Read the model definition and answer for the solid it produces. Units are mm, in the model's axes. A direction names the side the tool comes from. Give positions to 0.01 mm unless a question says otherwise; leave off trailing zeros. Order: outer loops, then holes, each group sorted by start corner. A loop starts at its lowest first (then second) coordinate and runs counter-clockwise, first axis right, second up.
Item 1: Find the intervals of material crossed by line 1 along Y through (x, z) = (0, -5.5); line 2 along Y through (x, z) = (-10.25, 0.75); line 3 along Z through (x, y) = (-2, 28), in increasing order.
Item 2: Given pin 1 Ø5 at (x, y) = (0, 39) entering from -Z; pin 2 Ø2 at (y, z) = (108.5, 8) entering from +X, each flat-ended and moving along its own axis, determine where each tip first touches the part or whether it passes through.
Item 3: A cutting plane is placed at A-A (x = 0). State how many separate pieces and enclosed holes the cut face has, plus the area to 3 significant figures.
Item 4: A cutting plane is placed at B-B (y = 39). Write down the section's boundary in (x, z).
Item 5: A cutting plane is placed at C-C (y = 309.5). Write down the section's boundary in (x, z), plus the area to 3 significant figures.
Item 6: Which of the six approach directions +Z, -Z, +X, -X, +Y, -Y give full straight-line access (tool end or side, diameter ignored) to faces 4 (the face through (0, 22, -1)), 5 (the face through (0, 0, -4))?
Item 7: The mould has two halves that part along Y. Classify faces 1 (the face through (-1, 173, 10.1)), 2 (the face through (0, 0, 4)), 3 (the face through (-0.521, 18.466, -5.486)): +Y half, -Y half, draft (parallel to the pull), parting line (faces both ways), or undercut.
from build123d import *

# Parameters (mm, degrees)
F0_W      = 30
F0_H      = 20.2
F1_DEPTH  = 350
F2_R      = 5
F3_R      = 3
F4_W      = 45.5
F4_H      = 2
F5_DEPTH  = 30.001
F6_W      = 5
F6_H      = 5
F7_DEPTH  = 30.001
F8_R      = 4
F9_DEPTH  = 20.201
F10_DEPTH = 30.001


with BuildPart() as f1:
    # F0 (on Front) → F1 (new body)
    with BuildSketch(Plane.XZ):
        Rectangle(F0_W, F0_H)
    extrude(amount=-F1_DEPTH)

    # F2
    f2_edges = [f1.edges().sort_by_distance(p)[0] for p in [
        (15, 175, 10.1),
    ]]
    fillet(f2_edges, radius=F2_R)

    # F3
    f3_edges = [f1.edges().sort_by_distance(p)[0] for p in [
        (-15, 175, 10.1),
        (-2.5, 0, 10.1),
        (-15, 175, -10.1),
        (15, 175, -10.1),
        (0, 0, -10.1),
        (0, 350, -10.1),
        (-15, 0, 0),
        (-2.5, 350, 10.1),
        (-15, 350, 0),
    ]]
    fillet(f3_edges, radius=F3_R)

    # F4 (on face) → F5 (cut, through all)
    with BuildSketch(Plane.YZ.offset(15)):
        with Locations((22.75, 0)):
            Rectangle(F4_W, F4_H)
    extrude(amount=-F5_DEPTH, mode=Mode.SUBTRACT)

    # F6 (on face) → F7 (cut, through all)
    with BuildSketch(Plane.YZ.offset(15)):
        with Locations((326, -1)):
            Rectangle(F6_W, F6_H)
    extrude(amount=-F7_DEPTH, mode=Mode.SUBTRACT)

    # F8 (on face) → F9 (cut, through all)
    with BuildSketch(Plane.XY.offset(10.1)):
        with Locations((0, 14.5)):
            Circle(F8_R)
        with Locations((0, 39)):
            Circle(F8_R)
    extrude(amount=-F9_DEPTH, mode=Mode.SUBTRACT)

    # F6 (on face) → F10 (cut, through all)
    with BuildSketch(Plane.YZ.offset(15)):
        with Locations((326, -1)):
            Rectangle(F6_W, F6_H)
    extrude(amount=-F10_DEPTH, mode=Mode.SUBTRACT)


solid = f1.part
Response values:
1. line 1: y = 0 to 10.5, 18.5 to 35, 43 to 350
1. line 2: y = 45.5 to 323.5, 328.5 to 350
1. line 3: z = -10.1 to -1, 1 to 10.1
2. pin 1: passes through
2. pin 2: stops at x = 14.62
3. separate pieces: 5
3. enclosed holes: 1
3. area: 6,660 mm2
4. outline: (-15, -7.1) arc R3 ccw to (-12, -10.1) - (-4, -10.1) - (-4, -1) - (-15, -1) - close; (-15, 1) - (-4, 1) - (-4, 10.1) - (-12, 10.1) arc R3 ccw to (-15, 7.1) - close; (4, -10.1) - (12, -10.1) arc R3 ccw to (15, -7.1) - (15, -1) - (4, -1) - close; (4, 1) - (15, 1) - (15, 5.1) arc R5 ccw to (10, 10.1) - (4, 10.1) - close
5. outline: (-15, -7.1) arc R3 ccw to (-12, -10.1) - (12, -10.1) arc R3 ccw to (15, -7.1) - (15, 5.1) arc R5 ccw to (10, 10.1) - (-12, 10.1) arc R3 ccw to (-15, 7.1) - close
5. area: 595 mm2
6. face 4: +X, -X, -Y
6. face 5: +Z, -Z, +X, -X, -Y
7. face 1: draft
7. face 2: -Y half
7. face 3: undercut
